Model file for the job. Use its own axes, mm. Face numbers are marked on the shaded views. A direction names the side the tool comes from. Round coordinates to 2 decimals unless told otherwise and drop trailing zeros. Loops run counter-clockwise (first coordinate to the right, second up) from the corner with the lowest first, then second, coordinate; pieces in that order, holes last. Notation, with made-up numbers: M -6,-18.5 L 49,-18.5 A24 ccw 49,-6.5 Z; hole C 70,13.5 d10. An arc over 180 degrees is marked long. Answer in a Markdown table with one row per item.
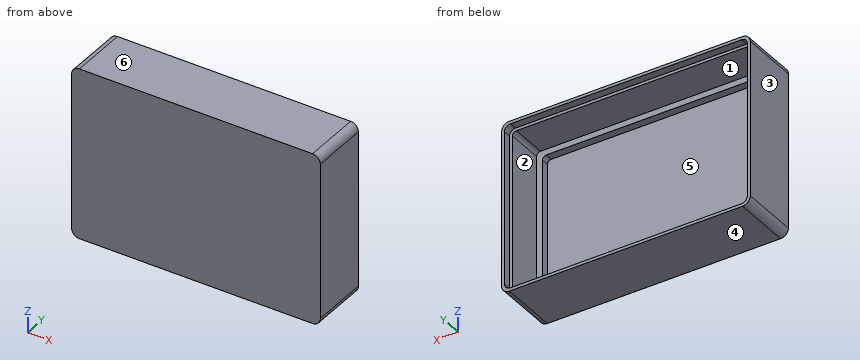
from build123d import *

# Parameters (mm, degrees)
SKETCH1_W           = 64
SKETCH1_H           = 44
BOSS_EXTRUDE1_DEPTH = 15
SKETCH2_W           = 61
SKETCH2_H           = 41
CUT_EXTRUDE1_DEPTH  = 13.5
SKETCH3_W           = 61
SKETCH3_H           = 41
SKETCH3_W_2         = 58
SKETCH3_H_2         = 38
BOSS_EXTRUDE2_DEPTH = 2
FILLET1_R           = 1
FILLET2_R           = 2
CUT_EXTRUDE2_DEPTH  = 2


with BuildPart() as part:
    # Sketch1 → Boss-Extrude1 (new body)
    with BuildSketch(Plane(origin=(0, 0, 0), x_dir=(1, 0, 0), z_dir=(0, 1, 0))):
        with Locations((32, 22)):
            Rectangle(SKETCH1_W, SKETCH1_H)
    extrude(amount=BOSS_EXTRUDE1_DEPTH)

    # Sketch2 → Cut-Extrude1 (cut)
    with BuildSketch(Plane(origin=(0, 15, 0), x_dir=(1, 0, 0), z_dir=(0, 1, 0))):
        with Locations((32, 22)):
            Rectangle(SKETCH2_W, SKETCH2_H)
    extrude(amount=-CUT_EXTRUDE1_DEPTH, mode=Mode.SUBTRACT)

    # Sketch3 → Boss-Extrude2 (add)
    with BuildSketch(Plane(origin=(0, 1.5, 0), x_dir=(1, 0, 0), z_dir=(0, 1, 0))):
        with Locations((32, 22)):
            Rectangle(SKETCH3_W, SKETCH3_H)
        with Locations((32.004099557, 22)):
            Rectangle(SKETCH3_W_2, SKETCH3_H_2, mode=Mode.SUBTRACT)
    extrude(amount=BOSS_EXTRUDE2_DEPTH)

    # Fillet1
    fillet1_edges = [part.edges().sort_by_distance(p)[0] for p in [
        (1.5, 9.25, -42.5),
        (62.5, 9.25, -42.5),
        (1.5, 9.25, -1.5),
        (62.5, 9.25, -1.5),
        (61.004099557, 2.5, -41),
        (3.004099557, 2.5, -41),
        (3.004099557, 2.5, -3),
        (61.004099557, 2.5, -3),
    ]]
    fillet(fillet1_edges, radius=FILLET1_R)

    # Fillet2
    fillet2_edges = [part.edges().sort_by_distance(p)[0] for p in [
        (0, 7.5, -44),
        (64, 7.5, -44),
        (64, 7.5, 0),
        (0, 7.5, 0),
    ]]
    fillet(fillet2_edges, radius=FILLET2_R)

    # Sketch4 → Cut-Extrude2 (cut)
    with BuildSketch(Plane(origin=(0, 15, 0), x_dir=(1, 0, 0), z_dir=(0, 1, 0))):
        with BuildLine():
            Line((2.25, 43.25), (61.75, 43.25))
            ThreePointArc((61.75, 43.25), (62.810660172, 42.810660172), (63.25, 41.75))
            Line((63.25, 41.75), (63.25, 2.25))
            ThreePointArc((63.25, 2.25), (62.810660172, 1.189339828), (61.75, 0.75))
            Line((61.75, 0.75), (2.25, 0.75))
            ThreePointArc((2.25, 0.75), (1.189339828, 1.189339828), (0.75, 2.25))
            Line((0.75, 2.25), (0.75, 41.75))
            ThreePointArc((0.75, 41.75), (1.189339828, 42.810660172), (2.25, 43.25))
        make_face()
        with BuildLine():
            Line((61.5, 42.5), (2.5, 42.5))
            ThreePointArc((2.5, 42.5), (1.792893219, 42.207106781), (1.5, 41.5))
            Line((1.5, 41.5), (1.5, 2.5))
            ThreePointArc((1.5, 2.5), (1.792893219, 1.792893219), (2.5, 1.5))
            Line((2.5, 1.5), (61.5, 1.5))
            ThreePointArc((61.5, 1.5), (62.207106781, 1.792893219), (62.5, 2.5))
            Line((62.5, 2.5), (62.5, 41.5))
            ThreePointArc((62.5, 41.5), (62.207106781, 42.207106781), (61.5, 42.5))
        make_face(mode=Mode.SUBTRACT)
    extrude(amount=-CUT_EXTRUDE2_DEPTH, mode=Mode.SUBTRACT)


solid = part.part
1. Saw through at A-A (y = 13.75). Write the cut outline in (x, z).
Verdict:
| item | result |
|---|---|
| outline | M 0,-42 A2 ccw 2,-44 L 62,-44 A2 ccw 64,-42 L 64,-2 A2 ccw 62,0 L 2,0 A2 ccw 0,-2 Z; hole M 0.75,-41.75 A1.5 ccw 2.25,-43.25 L 61.75,-43.25 A1.5 ccw 63.25,-41.75 L 63.25,-2.25 A1.5 ccw 61.75,-0.75 L 2.25,-0.75 A1.5 ccw 0.75,-2.25 Z |
2. Saw through at D-D (y = 7). Write the cut outline in (x, z), and give its area (3 significant figures).
Verdict:
| item | result |
|---|---|
| outline | M 0,-42 A2 ccw 2,-44 L 62,-44 A2 ccw 64,-42 L 64,-2 A2 ccw 62,0 L 2,0 A2 ccw 0,-2 Z; hole M 1.5,-41.5 A1 ccw 2.5,-42.5 L 61.5,-42.5 A1 ccw 62.5,-41.5 L 62.5,-2.5 A1 ccw 61.5,-1.5 L 2.5,-1.5 A1 ccw 1.5,-2.5 Z |
| area | 312 mm² |
3. Saw through at B-B (z = -38). Write the cut outline in (x, y), and give its area (4 significant figures).
Verdict:
| item | result |
|---|---|
| outline | M 0,0 L 64,0 L 64,15 L 63.25,15 L 63.25,13 L 62.5,13 L 62.5,3.5 L 61,3.5 L 61,1.5 L 3,1.5 L 3,3.5 L 1.5,3.5 L 1.5,13 L 0.75,13 L 0.75,15 L 0,15 Z |
| area | 139.5 mm² |
4. Pin check, flat tips, straight feed: pin 1 (4 mm diameter, centred on x = 13.5, z = -35, fed in from +Y); pin 2 (12 mm diameter, centred on x = 41, z = -7, fed in from +Y). Stop position of each tip, or through.
Verdict:
| item | result |
|---|---|
| pin 1 | stops at y = 1.5 |
| pin 2 | stops at y = 13 |
5. Mould opens along Z. For the marked faces 1, 2, 3 and 4 say: +Z half, -Z half, draft (parallel to the pull), parting line (faces both ways), or undercut.
Verdict:
| item | result |
|---|---|
| face 1 | undercut |
| face 2 | undercut |
| face 3 | draft |
| face 4 | -Z half |
6. Wall check: probe 1 along Z at (x, y) = (29, 8); probe 2 along X at (y, z) = (10.25, -7); probe 3 along Z at (x, y) = (32, 14). Give the ranges that are in metal, low to high.
Verdict:
| item | result |
|---|---|
| probe 1 | z = -44 to -42.5, -1.5 to 0 |
| probe 2 | x = 0 to 1.5, 62.5 to 64 |
| probe 3 | z = -44 to -43.25, -0.75 to 0 |
7. Saw through at C-C (x = 39). Write the cut outline in (y, z), and give its area (4 significant figures).
Verdict:
| item | result |
|---|---|
| outline | M 0,-44 L 15,-44 L 15,-43.25 L 13,-43.25 L 13,-42.5 L 3.5,-42.5 L 3.5,-41 L 1.5,-41 L 1.5,-3 L 3.5,-3 L 3.5,-1.5 L 13,-1.5 L 13,-0.75 L 15,-0.75 L 15,0 L 0,0 Z |
| area | 109.5 mm² |
8. Tool access for the marked faces 5 and 6: list every direction of +Z, -Z, +X, -X, +Y, -Y with a clear straight run to the whole face (end or side of a thin tool).
Verdict:
| item | result |
|---|---|
| face 5 | +Y |
| face 6 | +Z, +X, -X, +Y, -Y |
